Geometry: final body of the model. Coordinates: model frame, mm. Give positions to 0.01 mm unless a question says otherwise; leave off trailing zeros. Order: outer loops, then holes, each group sorted by start corner. A loop starts at its lowest first (then second) coordinate and runs counter-clockwise, first axis right, second up. Notation, with made-up numbers: (-34, 53) -> (18, 53) arc R36 ccw to (18, 87) -> close; hole circle Ø11 at (51, 30.5). An arc over 180 degrees is marked (long way). One line per question, with ' | ' between items.
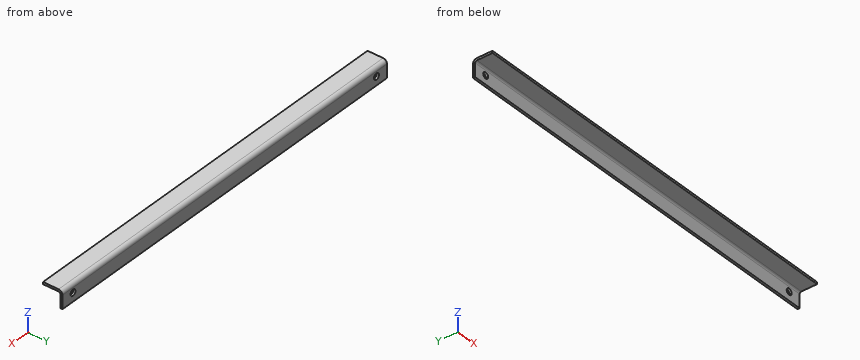
from build123d import *

# Parameters (mm, degrees)
SKETCH1_W           = 462.50664735
SKETCH1_H           = 20
BOSS_EXTRUDE1_DEPTH = 2.5
SKETCH2_R           = 3.5
CUT_EXTRUDE1_DEPTH  = 2.5
SKETCH3_W           = 462.50664735
SKETCH3_H           = 2.5
BOSS_EXTRUDE2_DEPTH = 20
FILLET1_R           = 2
FILLET2_R           = 4.5


with BuildPart() as part:
    # Sketch1 → Boss-Extrude1 (new body)
    with BuildSketch(Plane(origin=(0, 0, 0), x_dir=(1, 0, 0), z_dir=(0, 1, 0))):
        Rectangle(SKETCH1_W, SKETCH1_H)
    extrude(amount=BOSS_EXTRUDE1_DEPTH)

    # Sketch2 → Cut-Extrude1 (cut)
    with BuildSketch(Plane(origin=(0, 2.5, 0), x_dir=(1, 0, 0), z_dir=(0, 1, 0))):
        with Locations(Location((216.253323675, 0, 0), (0, 0, 270))):
            Circle(SKETCH2_R)
        with Locations(Location((-216.253323675, 0, 0), (0, 0, 270))):
            Circle(SKETCH2_R)
    extrude(amount=-CUT_EXTRUDE1_DEPTH, mode=Mode.SUBTRACT)

    # Sketch3 → Boss-Extrude2 (add)
    with BuildSketch(Plane.XZ):
        with Locations((0, 8.75)):
            Rectangle(SKETCH3_W, SKETCH3_H)
    extrude(amount=BOSS_EXTRUDE2_DEPTH)

    # Fillet1
    fillet1_edges = [part.edges().sort_by_distance(p)[0] for p in [
        (0, 0, 7.5),
    ]]
    fillet(fillet1_edges, radius=FILLET1_R)

    # Fillet2
    fillet2_edges = [part.edges().sort_by_distance(p)[0] for p in [
        (0, 2.5, 10),
    ]]
    fillet(fillet2_edges, radius=FILLET2_R)


solid = part.part
1) Section C-C on y = -16.5. Return loops of the section in (x, z).
Check result:
outline: (-231.25, 7.5) -> (231.25, 7.5) -> (231.25, 10) -> (-231.25, 10) -> close
2) Section B-B on x = -30.5. Return loops of the section in (y, z).
Check result:
outline: (-20, 7.5) -> (-2, 7.5) arc R2 cw to (0, 5.5) -> (0, -10) -> (2.5, -10) -> (2.5, 5.5) arc R4.5 ccw to (-2, 10) -> (-20, 10) -> close
3) Section A-A on z = 0. Return loops of the section in (x, y), plus the area to 3 significant figures.
Check result:
outline: (-231.25, 0) -> (-219.75, 0) -> (-219.75, 2.5) -> (-231.25, 2.5) -> close; (-212.75, 0) -> (212.75, 0) -> (212.75, 2.5) -> (-212.75, 2.5) -> close; (219.75, 0) -> (231.25, 0) -> (231.25, 2.5) -> (219.75, 2.5) -> close | area: 1,120 mm^2
4) Contact query for flat-ended pins moving along their axis: pin 1 Ø10 at (x, y) = (-106, -13) entering from -Z; pin 2 Ø10 at (y, z) = (-3.5, -7.5) entering from -X; pin 3 Ø11 at (x, z) = (216.25, 0) entering from -Y. Output: stop coordinate, or through.
Check result:
pin 1: stops at z = 7.5 | pin 2: stops at x = -231.25 | pin 3: stops at y = 0
5) Material intervals for probe 1 along X at (y, z) = (1.55, 0); probe 2 along Z at (x, y) = (-95.5, -10.75); probe 3 along Y at (x, z) = (-211, -6.5), sorted ascending. Write a range as from..to.
Check result:
probe 1: x = -231.25..-219.75, -212.75..212.75, 219.75..231.25 | probe 2: z = 7.5..10 | probe 3: y = 0..2.5
